from build123d import *

# Parameters (mm, degrees)
F0_W      = 46
F0_H      = 46
F1_DEPTH  = 2
F2_R      = 2
F3_DEPTH  = 25.4
F4_R      = 22.5
F5_DEPTH  = 20
F6_R      = 20
F7_DEPTH  = 16
F9_W      = 46
F9_H      = 46
F10_DEPTH = 2
F12_W     = 13
F12_H     = 3.5
F13_DEPTH = 4.7
F14_W     = 9
F14_H     = 4
F15_DEPTH = 2.7
F16_R     = 2
F17_DEPTH = 2
F18_R     = 2
F19_DEPTH = 2
F20_R     = 2
F21_DEPTH = 2


with BuildPart() as f1:
    # F0 (on Top) → F1 (new body)
    with BuildSketch(Plane.XY):
        with Locations((23, -23)):
            Rectangle(F0_W, F0_H)
    extrude(amount=F1_DEPTH)

    # F2 (on face) → F3 (cut)
    with BuildSketch(Plane.XY.offset(2)):
        with Locations((5.5, -5.5)):
            Circle(F2_R)
    extrude(amount=-F3_DEPTH, mode=Mode.SUBTRACT)

    # F4 (on face) → F5 (join)
    with BuildSketch(Plane(origin=(0, 0, 0), x_dir=(1, 0, 0), z_dir=(0, 0, -1))):
        with Locations((23, 23)):
            Circle(F4_R)
    extrude(amount=-F5_DEPTH)

    # F6 (on face) → F7 (cut, symmetric)
    with BuildSketch(Plane.XY.offset(2)):
        with Locations((23, -23)):
            Circle(F6_R)
    extrude(amount=F7_DEPTH, both=True, mode=Mode.SUBTRACT)

    # F9 (on offset) → F10 (join)
    with BuildSketch(Plane.XY.offset(18.7)):
        with Locations((23, -23)):
            Rectangle(F9_W, F9_H)
    extrude(amount=F10_DEPTH)

    # F12 (on face) → F13 (cut)
    with BuildSketch(Plane.XY.offset(20.7)):
        with Locations((21.5, -4.8802558407)):
            Rectangle(F12_W, F12_H)
    extrude(amount=-F13_DEPTH, mode=Mode.SUBTRACT)

    # F14 (on face) → F15 (cut)
    with BuildSketch(Plane.XY.offset(20.7)):
        with Locations((31.5, -35.4355278909)):
            Rectangle(F14_W, F14_H)
    extrude(amount=-F15_DEPTH, mode=Mode.SUBTRACT)

    # F16 (on face) → F17 (cut)
    with BuildSketch(Plane(origin=(0, 0, 0), x_dir=(1, 0, 0), z_dir=(0, 0, -1))):
        with Locations((40.5, 40.5)):
            Circle(F16_R)
    extrude(amount=-F17_DEPTH, mode=Mode.SUBTRACT)

    # F18 (on face) → F19 (cut)
    with BuildSketch(Plane(origin=(0, 0, 0), x_dir=(1, 0, 0), z_dir=(0, 0, -1))):
        with Locations((40.5, 5.5)):
            Circle(F18_R)
    extrude(amount=-F19_DEPTH, mode=Mode.SUBTRACT)

    # F20 (on face) → F21 (cut)
    with BuildSketch(Plane(origin=(0, 0, 0), x_dir=(1, 0, 0), z_dir=(0, 0, -1))):
        with Locations((5.5, 40.5)):
            Circle(F20_R)
    extrude(amount=-F21_DEPTH, mode=Mode.SUBTRACT)


solid = f1.part
Design review of the part built by this model. Coordinates are the model's own, in mm. A direction names the side the tool comes from. Coordinates: 2 decimals unless noted, no trailing zeros. Loops run counter-clockwise (first coordinate to the right, second up) from the corner with the lowest first, then second, coordinate; pieces in that order, holes last. Notation, with made-up numbers: M -39.5,55 L -21.5,55 A16 cw -21.5,72 Z; hole C 70.25,-9 d5. An arc over 180 degrees is marked long. Use one line per item in the form item = value.
(1) Draft analysis for pull direction Z (two halves, no side actions). For faces 5 (the face through (23, -23, 18)), 6 (the face through (2, -13, 18.7)), 7 (the face through (21.4, -3.13, 18.4)), state which applies: pulls with the +Z half, pulls with the -Z half, needs draft (parallel to the pull), parting line crosses it, or undercut.
Return value:
face_5 = pulls with the -Z half
face_6 = undercut
face_7 = needs draft
(2) For line 1 along X through (y, z) = (-23, 9.5); line 2 along Z through (x, y) = (37, -2); line 3 along Y through (x, z) = (40.5, 1.3), list the stretches that pass through material, from the lowest coordinate up. Write a range as from..to.
Return value:
line_1 = 0.5..3, 43..45.5
line_2 = 0..2, 18.7..20.7
line_3 = -46..-42.5, -38.5..-32.68, -13.32..-7.5, -3.5..0
(3) Clearance check with flat-ended pins moving along their axes: P1, Ø5, axis at y = -8, z = 11.5, coming from the +X side; P2, Ø1.5, axis at y = -22, z = 12, coming from the +X side; P3, Ø3, axis at x = 5.5, y = -5.5, coming from the -Z side. State where each tip first meets the part, or that it passes through.
Return value:
P1 = 41.71
P2 = 45.5
P3 = 18.7
(4) For faces 1 (the face through (5.145, -9.309, 10.233)), 2 (the face through (28, -5, 19)), 3 (the face through (3.9, -6.7, 1)), 4 (the face through (31, -33.436, 19)), list the 3-axis set-ups (+Z, -Z, +X, -X, +Y, -Y) from which the entire face can be reached by the end or side of a thin tool; tool diameter is ignored.
Return value:
face_1 = none
face_2 = +Z
face_3 = -Z
face_4 = +Z, -Z
(5) Consider section D-D (y = -23). Write out the cut boundary in (x, z).
Return value:
outline = M 0,0 L 3,0 L 3,18 L 43,18 L 43,0 L 46,0 L 46,2 L 45.5,2 L 45.5,18.7 L 46,18.7 L 46,20.7 L 0,20.7 L 0,18.7 L 0.5,18.7 L 0.5,2 L 0,2 Z
(6) Consider section A-A (x = 23). Write out the cut boundary in (y, z), and give its area (3 significant figures).
Return value:
outline = M -46,0 L -43,0 L -43,18 L -6.63,18 L -6.63,20.7 L -46,20.7 L -46,18.7 L -45.5,18.7 L -45.5,2 L -46,2 Z; M -3.13,18 L -3,18 L -3,0 L 0,0 L 0,2 L -0.5,2 L -0.5,18.7 L 0,18.7 L 0,20.7 L -3.13,20.7 Z
area = 206 mm2
(7) Consider section C-C (x = 5.5). Write out the cut boundary in (y, z), and give its area (3 significant figures).
Return value:
outline = M -46,0 L -42.5,0 L -42.5,2 L -46,2 Z; M -46,18.7 L -37.14,18.7 L -37.14,2 L -38.5,2 L -38.5,0 L -32.68,0 L -32.68,18 L -13.32,18 L -13.32,0 L -7.5,0 L -7.5,2 L -8.86,2 L -8.86,18.7 L 0,18.7 L 0,20.7 L -46,20.7 Z; M -3.5,0 L 0,0 L 0,2 L -3.5,2 Z
area = 292 mm2
(8) Consider section B-B (y = -36.5). Write out the cut boundary in (x, z), and give its area (3 significant figures).
Return value:
outline = M 0,0 L 8.24,0 L 8.24,18 L 27,18 L 27,20.7 L 0,20.7 L 0,18.7 L 5,18.7 L 5,2 L 0,2 Z; M 36,18 L 37.76,18 L 37.76,0 L 46,0 L 46,2 L 41,2 L 41,18.7 L 46,18.7 L 46,20.7 L 36,20.7 Z
area = 230 mm2
